Here's how the part is built. I have some questions about the finished solid (model axes, mm). Round coordinates to 2 decimals unless told otherwise and drop trailing zeros. Write each loop counter-clockwise with the first axis right and the second up, starting at its lowest first coordinate (ties: lowest second). Pieces come first, ordered by that corner, then holes. Notation, with made-up numbers: M 68.25,-31.5 L 108.25,-31.5 A19 cw 108.25,-15.5 Z; hole C -36.75,53 d4. An arc over 180 degrees is marked long. Use one line per item in the form item = value. Start each with the question number.
Q1. I want a section at B-B on z = 1. List the corners of the cut face in (x, y) for me, and give its area (3 significant figures).
Q2. I need wall thicknesses on line 1 along X through (y, z) = (6, -2); line 2 along X through (y, z) = (4.5, -2.5); line 3 along X through (y, z) = (1.5, -6). Which ranges of each line are inside material? Lowest first, please. Write a range as from..to.
Q3. I want a section at C-C on z = 6.25. List the corners of the cut face in (x, y) for me.
Q4. I'm going to push a flat-ended pin straight in: pin 1 Ø1 at (x, z) = (17.5, 6) entering from -Y. Where does the tip first touch, or does it pass through?
Q5. I want a section at A-A on y = 3.75. State how many separate pieces and enclosed holes the cut face has, and give its area (3 significant figures).
```python
from build123d import *

# Parameters (mm, degrees)
BOSS_EXTRUDE1_DEPTH = 9
FILLET1_R           = 7.5


with BuildPart() as part:
    # Sketch1 → Boss-Extrude1 (new body)
    with BuildSketch(Plane(origin=(0, 0, 0), x_dir=(1, 0, 0), z_dir=(0, 1, 0))):
        with BuildLine():
            Line((-50, 7.5), (-50, -7.5))
            Line((-50, -7.5), (-42.5, -7.5))
            Line((-42.5, -7.5), (-42.5, -3.175))
            ThreePointArc((-42.5, -3.175), (-45.675, 0), (-42.5, 3.175))
            Line((-42.5, 3.175), (-42.5, 7.5))
            Line((-42.5, 7.5), (-50, 7.5))
        make_face()
        with BuildLine():
            Line((-42.5, -3.175), (-42.5, -7.5))
            Line((-42.5, -7.5), (42.5, -7.5))
            Line((42.5, -7.5), (42.5, -3.175))
            ThreePointArc((42.5, -3.175), (39.325, 0), (42.5, 3.175))
            Line((42.5, 3.175), (42.5, 7.5))
            Line((42.5, 7.5), (-42.5, 7.5))
            Line((-42.5, 7.5), (-42.5, 3.175))
            ThreePointArc((-42.5, 3.175), (-40.25493597, 2.24506403), (-39.325, 0))
            ThreePointArc((-39.325, 0), (-40.25493597, -2.24506403), (-42.5, -3.175))
        make_face()
        with BuildLine():
            Line((42.5, -3.175), (42.5, -7.5))
            Line((42.5, -7.5), (50, -7.5))
            Line((50, -7.5), (50, 7.5))
            Line((50, 7.5), (42.5, 7.5))
            Line((42.5, 7.5), (42.5, 3.175))
            ThreePointArc((42.5, 3.175), (44.74506403, 2.24506403), (45.675, 0))
            ThreePointArc((45.675, 0), (44.74506403, -2.24506403), (42.5, -3.175))
        make_face()
    extrude(amount=BOSS_EXTRUDE1_DEPTH)

    # Fillet1
    fillet1_edges = [part.edges().sort_by_distance(p)[0] for p in [
        (50, 4.5, 7.5),
        (50, 4.5, -7.5),
        (-50, 4.5, 7.5),
        (-50, 4.5, -7.5),
    ]]
    fillet(fillet1_edges, radius=FILLET1_R - 0.0001)  # a hair under: the kernel refuses the full size


solid = part.part
```
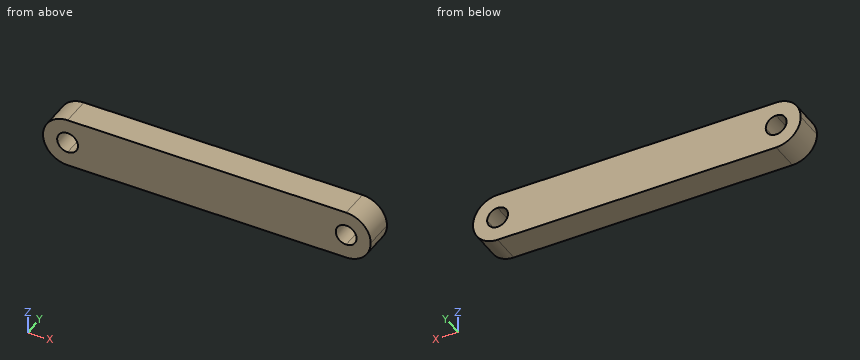
Reported:
q1.outline = M -49.93,0 L -45.51,0 L -45.51,9 L -49.93,9 Z; M -39.49,0 L 39.49,0 L 39.49,9 L -39.49,9 Z; M 45.51,0 L 49.93,0 L 49.93,9 L 45.51,9 Z
q1.area = 790 mm^2
q2.line_1 = -49.73..-44.97, -40.03..40.03, 44.97..49.73
q2.line_2 = -49.57..-44.46, -40.54..40.54, 44.46..49.57
q2.line_3 = -47..47
q3.outline = M -46.65,0 L 46.65,0 L 46.65,9 L -46.65,9 Z
q4.pin_1 = 0
q5.separate_pieces = 1
q5.enclosed_holes = 2
q5.area = 1,390 mm^2
